```python
from build123d import *

# Parameters (mm, degrees)
ESBO_O1_R                = 28.7
RESSALTO_EXTRUS_O1_DEPTH = 5
ESBO_O2_R                = 11
CORTE_EXTRUS_O1_DEPTH    = 8
ESBO_O3_R                = 7.5
CORTE_EXTRUS_O2_DEPTH    = 42.801674608
RESSALTO_EXTRUS_O4_START = 10
RESSALTO_EXTRUS_O4_DEPTH = 10
ESBO_O9_W                = 10
ESBO_O9_H                = 2
CORTE_EXTRUS_O5_DEPTH    = 10
CHANFRO1_SIZE            = 2
ESBO_O10_R               = 1.8
CORTE_EXTRUS_O6_DEPTH    = 10
CORTE_EXTRUS_O7_START    = -3
CORTE_EXTRUS_O7_DEPTH    = 2.9
CORTE_EXTRUS_O8_START    = -5
ESBO_O13_R               = 28.7
CORTE_EXTRUS_O8_DEPTH    = 5
ESBO_O14_R               = 28.7
ESBO_O14_R_2             = 26.2
CORTE_EXTRUS_O9_DEPTH    = 44.271006459
ESBO_O15_R               = 1.6
CORTE_EXTRUS_O10_DEPTH   = 40.973491216
CORTE_EXTRUS_O11_START   = -3
CORTE_EXTRUS_O11_DEPTH   = 42.378118766
RESSALTO_EXTRUS_O5_START = -5
RESSALTO_EXTRUS_O5_DEPTH = 5
ESBO_O19_W               = 22
ESBO_O19_H               = 15
RESSALTO_EXTRUS_O6_DEPTH = 5
FILETE1_R                = 3
FILETE2_R                = 1
FILETE3_R                = 1


with BuildPart() as part:
    # Esboço1 → Ressalto-extrusão1 (new, symmetric)
    with BuildSketch(Plane.XY):
        Circle(ESBO_O1_R)
    extrude(amount=RESSALTO_EXTRUS_O1_DEPTH, both=True)

    # Esboço2 → Corte-extrusão1 (cut)
    with BuildSketch(Plane.XY.offset(5)):
        Circle(ESBO_O2_R)
    extrude(amount=-CORTE_EXTRUS_O1_DEPTH, mode=Mode.SUBTRACT)

    # Esboço3 → Corte-extrusão2 (cut, through all)
    with BuildSketch(Plane(origin=(0, 0, -5), x_dir=(-1, 0, 0), z_dir=(0, 0, -1))):
        Circle(ESBO_O3_R)
    extrude(amount=-CORTE_EXTRUS_O2_DEPTH, mode=Mode.SUBTRACT)

    # Esboço8 → Ressalto-extrusão4 (add)
    with BuildSketch(Plane.XY.offset(5).offset(RESSALTO_EXTRUS_O4_START)):
        with BuildLine():
            Line((-11, 0), (-28.7, 0))
            ThreePointArc((-28.7, 0), (0, -28.7), (28.7, 0))
            Line((28.7, 0), (11, 0))
            ThreePointArc((11, 0), (0, -11), (-11, 0))
        make_face()
    extrude(amount=-RESSALTO_EXTRUS_O4_DEPTH)

    # Esboço9 → Corte-extrusão5 (cut)
    with BuildSketch(Plane.XY.offset(15)):
        with Locations((-19.85, -1)):
            Rectangle(ESBO_O9_W, ESBO_O9_H)
        with Locations((19.85, -1)):
            Rectangle(ESBO_O9_W, ESBO_O9_H)
    extrude(amount=-CORTE_EXTRUS_O5_DEPTH, mode=Mode.SUBTRACT)

    # Chanfro1
    chanfro1_edges = [part.edges().sort_by_distance(p)[0] for p in [
        (24.85, 0, 10),
        (14.85, 0, 10),
        (-14.85, 0, 10),
        (-24.85, 0, 10),
    ]]
    chamfer(chanfro1_edges, length=CHANFRO1_SIZE - 0.0001)  # a hair under: the kernel refuses the full size

    # Esboço10 → Corte-extrusão6 (cut)
    with BuildSketch(Plane(origin=(0, -2, 0), x_dir=(1, 0, 0), z_dir=(0, 1, 0))):
        with Locations(Location((-19.85, -10, 0), (0, 0, 180))):
            Circle(ESBO_O10_R)
        with Locations((19.85, -10)):
            Circle(ESBO_O10_R)
    extrude(amount=-CORTE_EXTRUS_O6_DEPTH, mode=Mode.SUBTRACT)

    # Esboço11 → Corte-extrusão7 (cut)
    with BuildSketch(Plane(origin=(0, -2, 0), x_dir=(1, 0, 0), z_dir=(0, 1, 0)).offset(CORTE_EXTRUS_O7_START)):
        Polygon((-23, -8.181346652), (-23, -11.818653348), (-23, -15), (-16.7, -15), (-16.7, -11.818653348), (-16.7, -8.181346652), (-19.85, -6.362693304), align=None)
        Polygon((23, -15), (23, -11.818653348), (23, -8.181346652), (19.85, -6.362693304), (16.7, -8.181346652), (16.7, -11.818653348), (16.7, -15), align=None)
    extrude(amount=-CORTE_EXTRUS_O7_DEPTH, mode=Mode.SUBTRACT)

    # Esboço13 → Corte-extrusão8 (cut)
    with BuildSketch(Plane(origin=(0, 0, -5), x_dir=(-1, 0, 0), z_dir=(0, 0, -1)).offset(CORTE_EXTRUS_O8_START)):
        Circle(ESBO_O13_R)
    extrude(amount=CORTE_EXTRUS_O8_DEPTH, mode=Mode.SUBTRACT)

    # Esboço14 → Corte-extrusão9 (cut, through all)
    with BuildSketch(Plane(origin=(0, 0, 0), x_dir=(-1, 0, 0), z_dir=(0, 0, -1))):
        Circle(ESBO_O14_R)
        Circle(ESBO_O14_R_2, mode=Mode.SUBTRACT)
    extrude(amount=-CORTE_EXTRUS_O9_DEPTH, mode=Mode.SUBTRACT)

    # Esboço15 → Corte-extrusão10 (cut, through all)
    with BuildSketch(Plane(origin=(0, 0, 0), x_dir=(-1, 0, 0), z_dir=(0, 0, -1))):
        with Locations((-12.374368671, 12.374368671)):
            Circle(ESBO_O15_R)
        with Locations((12.374368671, 12.374368671)):
            Circle(ESBO_O15_R)
        with Locations((12.374368671, -12.374368671)):
            Circle(ESBO_O15_R)
        with Locations((-12.374368671, -12.374368671)):
            Circle(ESBO_O15_R)
    extrude(amount=-CORTE_EXTRUS_O10_DEPTH, mode=Mode.SUBTRACT)

    # Esboço17 → Corte-extrusão11 (cut, through all)
    with BuildSketch(Plane.XY.offset(5).offset(CORTE_EXTRUS_O11_START)):
        Polygon((-15.524368671, 14.193022019), (-15.524368671, 10.555715323), (-12.374368671, 8.737061975), (-9.224368671, 10.555715323), (-9.224368671, 14.193022019), (-12.374368671, 16.011675367), align=None)
        Polygon((16.011675367, 12.374368671), (14.193022019, 15.524368671), (10.555715323, 15.524368671), (8.737061975, 12.374368671), (10.555715323, 9.224368671), (14.193022019, 9.224368671), align=None)
        Polygon((12.374368671, -16.011675367), (15.524368671, -14.193022019), (15.524368671, -10.555715323), (12.374368671, -8.737061975), (9.224368671, -10.555715323), (9.224368671, -14.193022019), align=None)
        Polygon((-16.011675367, -12.374368671), (-14.193022019, -15.524368671), (-10.555715323, -15.524368671), (-8.737061975, -12.374368671), (-10.555715323, -9.224368671), (-14.193022019, -9.224368671), align=None)
    extrude(amount=CORTE_EXTRUS_O11_DEPTH, mode=Mode.SUBTRACT)

    # Esboço18 → Ressalto-extrusão5 (add)
    with BuildSketch(Plane.XY.offset(5).offset(RESSALTO_EXTRUS_O5_START)):
        with BuildLine():
            Line((-2.5, 26.08045245), (-2.5, 46.08045245))
            Line((-2.5, 46.08045245), (2.5, 46.08045245))
            Line((2.5, 46.08045245), (2.5, 26.08045245))
            ThreePointArc((2.5, 26.08045245), (0, 26.2), (-2.5, 26.08045245))
        make_face()
    extrude(amount=RESSALTO_EXTRUS_O5_DEPTH)

    # Esboço19 → Ressalto-extrusão6 (add)
    with BuildSketch(Plane(origin=(2.5, 0, 0), x_dir=(0, 0, -1), z_dir=(1, 0, 0))):
        with Locations((11, 38.58045245)):
            Rectangle(ESBO_O19_W, ESBO_O19_H)
    extrude(amount=-RESSALTO_EXTRUS_O6_DEPTH)

    # Filete1
    filete1_edges = [part.edges().sort_by_distance(p)[0] for p in [
        (2.5, 26.08045245, 2.5),
        (-2.5, 26.08045245, 2.5),
    ]]
    fillet(filete1_edges, radius=FILETE1_R)

    # Filete2
    filete2_edges = [part.edges().sort_by_distance(p)[0] for p in [
        (0, 31.08045245, 0),
    ]]
    fillet(filete2_edges, radius=FILETE2_R)

    # Filete3
    filete3_edges = [part.edges().sort_by_distance(p)[0] for p in [
        (0, 46.08045245, 5),
        (0, 46.08045245, -22),
        (0, 31.08045245, -22),
    ]]
    fillet(filete3_edges, radius=FILETE3_R)


solid = part.part
```
Model file for the job. Use its own axes, mm. A direction names the side the tool comes from. Round coordinates to 2 decimals unless told otherwise and drop trailing zeros. Write each loop counter-clockwise with the first axis right and the second up, starting at its lowest first coordinate (ties: lowest second). Pieces come first, ordered by that corner, then holes. Notation, with made-up numbers: M -29,74 L -25,74 A25 ccw -25,99 Z; hole C 12.25,87 d7. An arc over 180 degrees is marked long. Put each result on its own line as item: value.
Item 1: Flat gauge pins, fed straight in: P1, Ø7, axis at x = 20, z = 12, coming from the +Y side; P2, Ø10, axis at x = 10.5, y = 37, coming from the +Z side; P3, Ø2, axis at x = 13, y = -10.5, coming from the -Z side; P4, Ø2.5, axis at x = 12, z = 3, coming from the -Y side. Where does each tip first touch, or does it go through?
Responses:
P1: y = -2
P2: through
P3: z = 0
P4: y = -23.89
Item 2: Probe L1, parallel to Z at x = 19.85, y = -10.65; L2, parallel to X at y = 34, z = 3; L3, parallel to Z at x = 5.5, y = 21. List the from-to ranges inside material, lowest first. Write a range as from..to.
Responses:
L1: 0..8.2, 11.8..15
L2: -2.5..2.5
L3: 0..5
Item 3: Tool access for faces 4 (the flat face through (20, -2, 8)), 5 (the flat face through (2.5, 38, -8)), 6 (the cylindrical face through (1.083, -26.178, 5.728)), 7 (the flat face through (15.09, 10.78, 3.48)): list every direction of +Z, -Z, +X, -X, +Y, -Y with a clear straight run to the whole face (end or side of a thin tool).
Responses:
face 4: +Z, +Y
face 5: +Z, -Z, +X, +Y
face 6: +Z, -Z
face 7: +Z
Item 4: Cut at D-D (x = -7.5). List the corners of the cut face in (y, z).
Responses:
outline: M -25.1,0 L -8.05,0 L -8.05,15 L -25.1,15 Z; M 8.05,0 L 25.1,0 L 25.1,5 L 8.05,5 Z
Item 5: Cut at A-A (x = 0). List the corners of the cut face in (y, z), and give its area (3 significant figures).
Responses:
outline: M -26.2,0 L -11,0 L -11,15 L -26.2,15 Z; M 11,0 L 30.08,0 A1 cw 31.08,-1 L 31.08,-21 A1 ccw 32.08,-22 L 45.08,-22 A1 ccw 46.08,-21 L 46.08,4 A1 ccw 45.08,5 L 11,5 Z
area: 733 mm²
Item 6: Cut at B-B (y = 7). List the corners of the cut face in (x, z).
Responses:
outline: M -25.25,0 L -8.49,0 L -8.49,5 L -25.25,5 Z; M 8.49,0 L 25.25,0 L 25.25,5 L 8.49,5 Z
Item 7: Mould opens along Z. For faces 1 (the flat face through (21.447, -6.43, 7.285)), 2 (the cylindrical face through (-21.513, -3.479, 9.311)), 3 (the flat face through (-12, -15.524, 8)) say: +Z half, -Z half, draft (parallel to the pull), parting line (faces both ways), or undercut.
Responses:
face 1: +Z half
face 2: undercut
face 3: draft
Item 8: Cut at C-C (z = 10). State how many separate pieces and enclosed holes the cut face has, and give its area (3 significant figures).
Responses:
separate pieces: 1
enclosed holes: 2
area: 684 mm²
